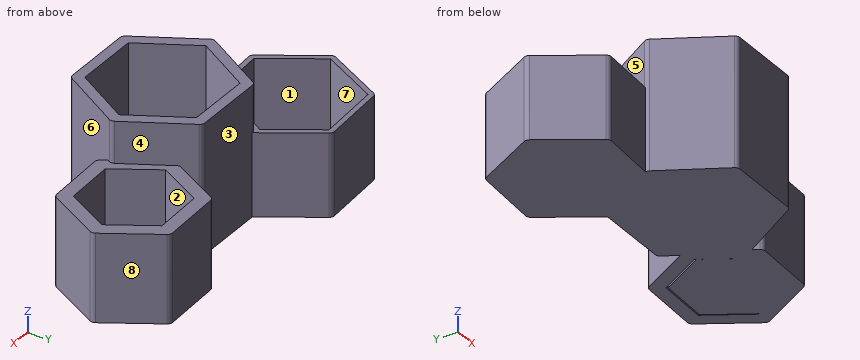
```python
from build123d import *

# Parameters (mm, degrees)
F1_DEPTH  = 100
F3_DEPTH  = 90
F4_DEPTH  = 25
F5_R      = 5
F7_DEPTH  = 25
F8_DEPTH  = 60
F9_R      = 5
F11_DEPTH = 10
F12_DEPTH = 50
F14_DEPTH = 10
F16_DEPTH = 80
F18_DEPTH = 75
F19_R     = 5


with BuildPart() as f1:
    # F0 (on Top) → F1 (new body)
    with BuildSketch(Plane.XY):
        Polygon((36.954793705, 64.0075802803), (-36.954793705, 64.0075802803), (-73.90958741, 0), (-36.954793705, -64.0075802803), (36.954793705, -64.0075802803), (73.90958741, 0), align=None)
    extrude(amount=F1_DEPTH)

    # F2 (on face) → F3 (cut)
    with BuildSketch(Plane.XY.offset(100)):
        Polygon((31.1812910131, 54.0075802803), (-31.1812910131, 54.0075802803), (-62.3625820262, 0), (-31.1812910131, -54.0075802803), (31.1812910131, -54.0075802803), (62.3625820262, 0), align=None)
    extrude(amount=-F3_DEPTH, mode=Mode.SUBTRACT)

    # F4 (add): a face of the model
    f4_faces = [f1.faces().sort_by_distance(p)[0] for p in [
        (53.7387091631, 31.0260582012, 100),
    ]]
    extrude(f4_faces, amount=F4_DEPTH)

    # F5
    f5_edges = [f1.edges().sort_by_distance(p)[0] for p in [
        (36.954794, -64.00758, 62.5),
        (73.909587, 0, 62.5),
        (36.954794, 64.00758, 62.5),
        (-36.954794, -64.00758, 62.5),
        (-73.909587, 0, 62.5),
        (-36.954794, 64.00758, 62.5),
    ]]
    fillet(f5_edges, radius=F5_R)

    # F6 (on Top) → F7 (join)
    with BuildSketch(Plane.XY):
        Polygon((72.4010563695, 97.2648855515), (42.7573003567, 41.3652363949), (76.3459385825, -12.2568339541), (139.5783328212, -9.9792551465), (169.222088834, 45.9203940101), (135.6334506082, 99.5424643591), align=None)
        Polygon((57.6229365769, 41.9006843788), (80.2975860361, 84.6585909333), (128.6643440546, 86.400721757), (154.3564526138, 45.3849460261), (131.6818031546, 2.6270394716), (83.3150451361, 0.884908648), align=None, mode=Mode.SUBTRACT)
    extrude(amount=F7_DEPTH)

    # F8 (add): a face of the model
    f8_faces = [f1.faces().sort_by_distance(p)[0] for p in [
        (104.0770804564, 96.7426995418, 25),
    ]]
    extrude(f8_faces, amount=F8_DEPTH)

    # F9
    f9_edges = [f1.edges().sort_by_distance(p)[0] for p in [
        (139.578333, -9.979255, 42.5),
        (169.222089, 45.920394, 42.5),
        (135.633451, 99.542464, 42.5),
        (76.345939, -12.256834, 42.5),
        (72.401056, 97.264886, 42.5),
    ]]
    fillet(f9_edges, radius=F9_R)

    # F13 (on Top) → F14 (join)
    with BuildSketch(Plane.XY):
        Polygon((80.7393563532, 83.0987106545), (58.3791809535, 40.7320548312), (83.8896934701, 0.1842469904), (131.7603813863, 2.0030949728), (154.120556786, 44.3697507961), (128.6100442695, 84.917558637), align=None)
    extrude(amount=F14_DEPTH)

    # F15 (on Top) → F16 (join)
    with BuildSketch(Plane.XY):
        Polygon((-62.4931809091, 1.7224331433), (-32.4628147698, 61.7831568187), (-69.4617441727, 117.8205786179), (-136.4910397149, 113.7972767418), (-166.5214058542, 53.7365530664), (-129.5224764513, -2.3008687328), align=None)
    extrude(amount=F16_DEPTH)

    # F17 (on face) → F18 (cut)
    with BuildSketch(Plane.XY.offset(80)):
        with BuildLine():
            Line((-72.0437333661, 112.6566009709), (-133.3098984847, 108.9792196846))
            Line((-133.3098984847, 108.9792196846), (-160.7582754306, 54.0824736562))
            Line((-160.7582754306, 54.0824736562), (-126.9404872579, 2.8631089142))
            Line((-126.9404872579, 2.8631089142), (-76.2742702816, 5.9042491226))
            Line((-76.2742702816, 5.9042491226), (-42.7282963969, 64.0075802803))
            ThreePointArc((-42.7282963969, 64.0075802803), (-42.0407030657, 65.043860696), (-41.2297996458, 65.986780275))
            Line((-41.2297996458, 65.986780275), (-72.0437333661, 112.6566009709))
        make_face()
    extrude(amount=-F18_DEPTH, mode=Mode.SUBTRACT)

    # F19
    f19_edges = [f1.edges().sort_by_distance(p)[0] for p in [
        (-129.522476, -2.300869, 40),
        (-166.521406, 53.736553, 40),
        (-136.49104, 113.797277, 40),
        (-69.461744, 117.820579, 40),
    ]]
    fillet(f19_edges, radius=F19_R)


with BuildPart() as f11:
    # F10 (on face) → F11 (new body)
    with BuildSketch(Plane.XY.offset(85)):
        Polygon((80.2975860361, 84.6585909333), (57.6229365769, 41.9006843788), (83.3150451361, 0.884908648), (131.6818031546, 2.6270394716), (154.3564526138, 45.3849460261), (128.6643440546, 86.400721757), align=None)
    extrude(amount=F11_DEPTH)

    # F12 (cut): a face of the model
    f12_faces = [f11.faces().sort_by_distance(p)[0] for p in [
        (105.9896945953, 43.6428152025, 95),
    ]]
    extrude(f12_faces, amount=-F12_DEPTH, mode=Mode.SUBTRACT)


solid = f1.part
```
CAD build for the part. Positions are in the model's coordinates, mm. Face numbers are marked on the shaded views. A direction names the side the tool comes from. Coordinates: 2 decimals unless noted, no trailing zeros. Order: outer loops, then holes, each group sorted by start corner. A loop starts at its lowest first (then second) coordinate and runs counter-clockwise, first axis right, second up.
(1) Saw through at D-D, the plane x = 2. Write the cut outline in (y, z).
Solution:
outline: (-64.01, 0) - (64.01, 0) - (64.01, 125) - (54.01, 125) - (54.01, 10) - (-54.01, 10) - (-54.01, 125) - (-64.01, 125) - close
(2) Pin check, flat tips, straight feed: pin 1 Ø3 at (x, z) = (-77, 76) entering from +Y; pin 2 Ø4 at (x, z) = (-54.5, 45.5) entering from -Y; pin 3 Ø2 at (x, y) = (-97, 68) entering from +Z. Stop position of each tip, or through.
Solution:
pin 1: stops at y = 117.46
pin 2: stops at y = -37.08
pin 3: stops at z = 5
(3) Saw through at C-C, the plane x = 66. Write the cut outline in (y, z).
Solution:
outline: (-13.7, 0) - (28.53, 0) - (28.53, 85) - (13.7, 85) - (13.7, 125) - (-13.7, 125) - close; (28.62, 0) - (55.17, 0) - (55.17, 10) - (28.62, 10) - close; (57.7, 0) - (85.19, 0) - (85.19, 85) - (57.7, 85) - close
(4) Which spindle directions (+Z, -Z, +X, -X, +Y, -Y) get a long thin tool onto all of the face, cutting with end or side? Do the marked faces 1, 2, 3, 4 and 5. Say none if no direction does.
Solution:
face 1: +Z
face 2: +Z, -Z
face 3: +Z, -Z, +Y
face 4: +Z, +Y
face 5: +Z, -X, +Y
(5) Saw through at A-A, the plane z = 100.5. Write the cut outline in (x, y).
Solution:
outline: (-72.47, -2.5) - (-38.4, -61.51) arc R5 ccw to (-34.07, -64.01) - (34.07, -64.01) arc R5 ccw to (38.4, -61.51) - (72.47, -2.5) arc R5 ccw to (72.47, 2.5) - (38.4, 61.51) arc R5 ccw to (34.07, 64.01) - (-34.07, 64.01) arc R5 ccw to (-38.4, 61.51) - (-72.47, 2.5) arc R5 ccw to start; hole (-62.36, 0) - (-31.18, -54.01) - (31.18, -54.01) - (62.36, 0) - (31.18, 54.01) - (-31.18, 54.01) - close
(6) Mould opens along Y. For the marked faces 6, 7 and 8 say: released by +Y, released by -Y, zero draft, split by the parting line, or undercut.
Solution:
face 6: released by -Y
face 7: undercut
face 8: released by +Y
(7) Saw through at B-B, the plane x = 104. Write the cut outline in (y, z), and give its area (3 significant figures).
Solution:
outline: (-11.26, 0) - (83.98, 0) - (83.98, 10) - (1.63, 10) - (1.63, 85) - (-11.26, 85) - close; (85.51, 0) - (98.4, 0) - (98.4, 85) - (85.51, 85) - close
area: 3,010 mm2
(8) Drill centre lines: L1, parallel to X at y = 41.5, z = 49.5; L2, parallel to X at y = 38, z = 15; L3, parallel to Y at x = 24, z = 47.5. Where is each one in solid material? Low to high.
Solution:
L1: x = -158.44 to -152.45, -55.72 to -38.4, 38.4 to 57.87, 152.3 to 166.88
L2: x = -156.13 to -150.14, -57.74 to -40.42, 40.42 to 60.07, 150.44 to 165.02
L3: y = -64.01 to -54.01, 54.01 to 64.01
